Read the model definition and answer for the solid it produces. Units are mm, in the model's axes. A direction names the side the tool comes from. Round coordinates to 2 decimals unless told otherwise and drop trailing zeros. Order: outer loops, then holes, each group sorted by start corner. A loop starts at its lowest first (then second) coordinate and runs counter-clockwise, first axis right, second up. Notation, with made-up numbers: (9.5, 7.5) - (52.5, 7.5) arc R26 ccw to (52.5, 36.5) - close; hole circle Ø1 at (-21.5, 22.25). An arc over 180 degrees is marked (long way). One line per question, with ' | ' between items. Start each with the question number.
1) The part is cut by section B-B, the plane z = 4.25. Give the vertices of the cut face in (x, y).
2) Flat-ended cylindrical pins translate along their axes: pin 1 (2 mm diameter, centred on x = 45, z = 1.5, fed in from -Y); pin 2 (0.6 mm diameter, centred on y = -15.5, z = 1.5, fed in from -X); pin 3 (1 mm diameter, centred on x = 44.5, z = 2.5, fed in from +Y); pin 4 (5 mm diameter, centred on x = 13, y = -7.5, fed in from -Z). Find the tip coordinate at first contact, or state that the pin passes through.
3) The part is cut by section C-C, the plane y = -12.75. Give the vertices of the cut face in (x, z), plus the area to 3 significant figures.
4) For faces 1 (the flat face through (44, -9.127, 2)), 2 (the flat face through (33.768, -12, 12)), 3 (the flat face through (45, -10, 5)), 4 (the flat face through (38, -14.925, 12)), 5 (the flat face through (45, -11.127, 2)), determine the directions among +Z, -Z, +X, -X, +Y, -Y from which every point of the face is accessible in a straight line to the end or side of a thin tool.
5) Straight lines are drawn through the part: line 1 (Z direction, x = 40, y = -15); line 2 (X direction, y = -5, z = 4); line 3 (Y direction, x = 36, z = 11.75). For each, find the intervals that lie inside material, in ascending order. Write a range as from..to.
6) The part is cut by section A-A, the plane x = 38. Give the vertices of the cut face in (y, z), plus the area to 3 significant figures.
7) The part is cut by section D-D, the plane z = 8. Give the vertices of the cut face in (x, y), plus the area to 3 significant figures.
8) The mould has two halves that part along X. Classify faces 6 (the flat face through (44, -15.127, 2)), 7 (the cylindrical face through (9.246, -2.981, 5.07)), 8 (the flat face through (47.326, -14, 2)): pulls with the +X half, pulls with the -X half, needs draft (parallel to the pull), parting line crosses it, or undercut.
from build123d import *

# Parameters (mm, degrees)
F1_DEPTH = 10
F2_DEPTH = 15
F3_R     = 3
F0_W     = 2
F0_H     = 2
F4_DEPTH = 5


with BuildPart() as f1:
    # F0 (on Top) → F1 (new body)
    with BuildSketch(Plane.XY):
        with BuildLine():
            Line((43.3439803123, -2.1253142133), (8.3439803123, -2.1253142133))
            Line((8.3439803123, -2.1253142133), (8.3439803123, -6.1607846163))
            ThreePointArc((8.3439803123, -6.1607846163), (13.9120945643, -7.088784926), (16.4613010362, -12.1253142133))
            ThreePointArc((16.4613010362, -12.1253142133), (13.9120945643, -17.1618435006), (8.3439803123, -18.0898438104))
            Line((8.3439803123, -18.0898438104), (8.3439803123, -22.1253142133))
            Line((8.3439803123, -22.1253142133), (43.3439803123, -22.1253142133))
            Line((43.3439803123, -22.1253142133), (43.3439803123, -15.1270665228))
            Line((43.3439803123, -15.1270665228), (43.3439803123, -14.9253142133))
            Line((43.3439803123, -14.9253142133), (33.7679572403, -14.9253142133))
            Line((33.7679572403, -14.9253142133), (33.7679572403, -9.3253142133))
            Line((33.7679572403, -9.3253142133), (43.3439803123, -9.3253142133))
            Line((43.3439803123, -9.3253142133), (43.3439803123, -9.1270665228))
            Line((43.3439803123, -9.1270665228), (43.3439803123, -2.1253142133))
        make_face()
        Polygon((43.3439803123, -11.1270665228), (43.3439803123, -9.3253142133), (33.7679572403, -9.3253142133), (33.7679572403, -14.9253142133), (43.3439803123, -14.9253142133), (43.3439803123, -13.1270665228), align=None)
    extrude(amount=F1_DEPTH)

    # F0 (on Top) → F2 (join)
    with BuildSketch(Plane.XY):
        Polygon((43.3439803123, -11.1270665228), (43.3439803123, -9.3253142133), (33.7679572403, -9.3253142133), (33.7679572403, -14.9253142133), (43.3439803123, -14.9253142133), (43.3439803123, -13.1270665228), align=None)
    extrude(amount=F2_DEPTH)

    # F3
    f3_edges = [f1.edges().sort_by_distance(p)[0] for p in [
        (8.34398, -22.125314, 5),
        (43.34398, -22.125314, 5),
        (43.34398, -2.125314, 5),
        (8.34398, -2.125314, 5),
    ]]
    fillet(f3_edges, radius=F3_R)

    # F0 (on Top) → F4 (join)
    with BuildSketch(Plane.XY):
        Polygon((45.3259829879, -9.1270665228), (43.3439803123, -9.1270665228), (43.3439803123, -9.3253142133), (43.3439803123, -11.1270665228), (44.0259829879, -11.1270665228), (45.3259829879, -11.1270665228), align=None)
        with Locations((46.3259829879, -10.1270665228)):
            Rectangle(F0_W, F0_H)
        Polygon((45.3259829879, -8.3770665228), (45.3259829879, -9.1270665228), (47.3259829879, -9.1270665228), align=None)
        with Locations((46.3259829879, -14.1270665228)):
            Rectangle(F0_W, F0_H)
        Polygon((47.3259829879, -15.1270665228), (45.3259829879, -15.1270665228), (45.3259829879, -15.8770665228), align=None)
        Polygon((44.0259829879, -13.1270665228), (43.3439803123, -13.1270665228), (43.3439803123, -14.9253142133), (43.3439803123, -15.1270665228), (45.3259829879, -15.1270665228), (45.3259829879, -13.1270665228), align=None)
    extrude(amount=F4_DEPTH)


solid = f1.part
Values:
1) outline: (8.34, -19.13) arc R3 ccw to (11.34, -22.13) - (40.34, -22.13) arc R3 ccw to (43.34, -19.13) - (43.34, -15.13) - (45.33, -15.13) - (45.33, -15.88) - (47.33, -15.13) - (47.33, -13.13) - (43.34, -13.13) - (43.34, -11.13) - (47.33, -11.13) - (47.33, -9.13) - (45.33, -8.38) - (45.33, -9.13) - (43.34, -9.13) - (43.34, -5.13) arc R3 ccw to (40.34, -2.13) - (11.34, -2.13) arc R3 ccw to (8.34, -5.13) - (8.34, -6.16) arc R6.25 cw (long way) to (8.34, -18.09) - close
2) pin 1: stops at y = -15.88 | pin 2: stops at x = 15.27 | pin 3: stops at y = -9.13 | pin 4: stops at z = 0
3) outline: (16.43, 0) - (43.34, 0) - (43.34, 15) - (33.77, 15) - (33.77, 10) - (16.43, 10) - close | area: 317 mm^2
4) face 1: +Z, -Z, +Y | face 2: +Z, -X, +Y, -Y | face 3: +Z, +X, +Y, -Y | face 4: +Z, +X, -X, -Y | face 5: +Z, -Z, +X
5) line 1: z = 0..10 | line 2: x = 8.35..43.34 | line 3: y = -14.93..-9.33
6) outline: (-22.13, 0) - (-2.13, 0) - (-2.13, 10) - (-9.33, 10) - (-9.33, 15) - (-14.93, 15) - (-14.93, 10) - (-22.13, 10) - close | area: 228 mm^2
7) outline: (8.34, -19.13) arc R3 ccw to (11.34, -22.13) - (40.34, -22.13) arc R3 ccw to (43.34, -19.13) - (43.34, -5.13) arc R3 ccw to (40.34, -2.13) - (11.34, -2.13) arc R3 ccw to (8.34, -5.13) - (8.34, -6.16) arc R6.25 cw (long way) to (8.34, -18.09) - close | area: 608 mm^2
8) face 6: undercut | face 7: pulls with the -X half | face 8: pulls with the +X half
